Geometry check sheet. Reference: the model listing, model coordinates, mm. A direction names the side the tool comes from. Coordinates: 2 decimals unless noted, no trailing zeros. Order: outer loops, then holes, each group sorted by start corner. A loop starts at its lowest first (then second) coordinate and runs counter-clockwise, first axis right, second up. Notation, with made-up numbers: (-18.75, -36.5) - (-2.75, -36.5) arc R9 ccw to (-2.75, -21.5) - close; hole circle Ø10 at (-6.75, 15). An arc over 180 degrees is marked (long way). Use CSV: the item, a comma, the result in double quotes. Start each with the question number.
1) Draft check along X on faces 4 (the flat face through (49, 15.1, -5.4)), 5 (the cylindrical face through (21.657, 2.465, 3.02)), 6 (the flat face through (-1, 5, 3)). Enter one of: released by +X, released by -X, zero draft, split by the parting line, or undercut.
2) Sectioned sample at A-A, the plane x = 39.5. Record the cut outline in (y, z).
3) Sectioned sample at B-B, the plane z = 2.5. Record the cut outline in (x, y), and give its area (3 significant figures).
4) Tool access check on faces 1 (the cylindrical face through (38.21, 7.07, -7.54)), 2 (the flat face through (-1, 23, -5)), 3 (the flat face through (-49, 15.1, -5.4)). Record the directions out of +Z, -Z, +X, -X, +Y, -Y that give a thin tool (end or side, any length) a straight path to the whole face; none if there is none.
5) Sectioned sample at D-D, the plane y = 20. Record the cut outline in (x, z).
6) Sectioned sample at C-C, the plane x = 24. Record the cut outline in (y, z), and give its area (3 significant figures).
7) Depth check by flat-ended pin: P1, Ø1.6, axis at x = 39.5, y = 36.9, coming from the -Z side; P2, Ø12, axis at y = 6, z = 3, coming from the -X side; P3, Ø3, axis at x = 10.5, z = 1.5, coming from the +Y side; P4, Ø12, axis at x = -21, y = 18.5, coming from the +Z side. Enter the tip coordinate at first touch or a pass-through.
8) Thickness scan on probe 1 along X at (y, z) = (3.5, 2.5); probe 2 along Y at (x, z) = (39.5, -7.35); probe 3 along Z at (x, y) = (12.5, 23.5). Record the ranges inside material, lowest first. Write a range as [from, to].
from build123d import *

# Parameters (mm, degrees)
SKETCH1_W                     = 98
SKETCH1_H                     = 20
BOSS_EXTRUDE1_DEPTH           = 5
SKETCH2_W                     = 98
SKETCH2_H                     = 5
BOSS_EXTRUDE2_DEPTH           = 35
FILLET1_R                     = 1
SKETCH5_W                     = 1.3
SKETCH5_H                     = 5
M2_CLEARANCE_HOLE1_AT_2_COUNT = 2
M2_CLEARANCE_HOLE1_AT_2_PITCH = 30
M2_CLEARANCE_HOLE1_AT_3_COUNT = 2
M2_CLEARANCE_HOLE1_AT_3_PITCH = 79
M2_CLEARANCE_HOLE1_AT_4_COUNT = 2
M2_CLEARANCE_HOLE1_AT_4_PITCH = 84.504437753
M4_CLEARANCE_HOLE1_D          = 4.8


with BuildPart() as part:
    # Sketch1 → Boss-Extrude1 (new body)
    with BuildSketch(Plane(origin=(0, 0, 0), x_dir=(1, 0, 0), z_dir=(0, 1, 0))):
        Rectangle(SKETCH1_W, SKETCH1_H)
    extrude(amount=BOSS_EXTRUDE1_DEPTH)

    # Sketch2 → Boss-Extrude2 (add)
    with BuildSketch(Plane(origin=(0, 5, 0), x_dir=(1, 0, 0), z_dir=(0, 1, 0))):
        with Locations((0, 7.5)):
            Rectangle(SKETCH2_W, SKETCH2_H)
    extrude(amount=BOSS_EXTRUDE2_DEPTH)

    # Fillet1
    fillet1_edges = [part.edges().sort_by_distance(p)[0] for p in [
        (0, 5, -5),
        (49, 40, -7.5),
        (-49, 40, -7.5),
        (0, 0, -10),
        (49, 2.5, 10),
        (-49, 2.5, 10),
    ]]
    fillet(fillet1_edges, radius=FILLET1_R)

    # Sketch5 → M2 Clearance Hole1 (revolve, cut)
    with BuildSketch(Plane(origin=(39.5, 36.904051391, -5), x_dir=(0, -1, 0), z_dir=(1, 0, 0))):
        with Locations((0.65, 2.5)):
            Rectangle(SKETCH5_W, SKETCH5_H)
    m2_clearance_hole1 = revolve(axis=Axis((39.5, 36.904051391, 1.35), (0, 0, -1)), mode=Mode.SUBTRACT)

    # M2 Clearance Hole1 at 2: M2 Clearance Hole1 ×2
    with Locations(*[(0, -i * M2_CLEARANCE_HOLE1_AT_2_PITCH, 0) for i in range(1, M2_CLEARANCE_HOLE1_AT_2_COUNT)]):
        add(m2_clearance_hole1, mode=Mode.SUBTRACT)

    # M2 Clearance Hole1 at 3: M2 Clearance Hole1 ×2
    with Locations(*[(-i * M2_CLEARANCE_HOLE1_AT_3_PITCH, 0, 0) for i in range(1, M2_CLEARANCE_HOLE1_AT_3_COUNT)]):
        add(m2_clearance_hole1, mode=Mode.SUBTRACT)

    # M2 Clearance Hole1 at 4: M2 Clearance Hole1 ×2
    with Locations(*[Vector(-0.93486214570929, -0.35501094140860234, 0) * (i * M2_CLEARANCE_HOLE1_AT_4_PITCH) for i in range(1, M2_CLEARANCE_HOLE1_AT_4_COUNT)]):
        add(m2_clearance_hole1, mode=Mode.SUBTRACT)

    # M4 Clearance Hole1 (through all)
    with Locations(Plane(origin=(-24, 5, 2.5), x_dir=(0, 0, 1), z_dir=(0, 1, 0))):
        with Locations((0, 0), (0, 48)):
            Hole(M4_CLEARANCE_HOLE1_D / 2)


solid = part.part
Evaluation:
1,face 4,"released by +X"
1,face 5,"undercut"
1,face 6,"zero draft"
2,outline,"(0, -9) arc R1 ccw to (1, -10) - (5.6, -10) - (5.6, -5) - (6, -5) arc R1 cw to (5, -4) - (5, 10) - (0, 10) - close; (8.2, -10) - (35.6, -10) - (35.6, -5) - (8.2, -5) - close; (38.2, -10) - (40, -10) - (40, -5) - (38.2, -5) - close"
3,outline,"(-49, 0) - (-26.4, 0) - (-26.4, 5) - (-49, 5) - close; (-21.6, 0) - (21.6, 0) - (21.6, 5) - (-21.6, 5) - close; (26.4, 0) - (49, 0) - (49, 5) - (26.4, 5) - close"
3,area,"442 mm²"
4,face 1,"-Z"
4,face 2,"+Z, +X, -X, +Y"
4,face 3,"+Z, -Z, -X, +Y, -Y"
5,outline,"(-49, -10) - (49, -10) - (49, -5) - (-49, -5) - close"
6,outline,"(0, -9) arc R1 ccw to (1, -10) - (40, -10) - (40, -5) - (6, -5) arc R1 cw to (5, -4) - (5, 0.1) - (0, 0.1) - close; (0, 4.9) - (5, 4.9) - (5, 10) - (0, 10) - close"
6,area,"251 mm²"
7,P1,"through"
7,P2,"x = -49"
7,P3,"y = 5"
7,P4,"z = -5"
8,probe 1,"[-49, -26.4], [-21.6, 21.6], [26.4, 49]"
8,probe 2,"[0, 5.6], [8.2, 35.6], [38.2, 40]"
8,probe 3,"[-10, -5]"
